Part model, mm, in its own coordinate system. Face numbers are marked on the shaded views. A direction names the side the tool comes from. Round coordinates to 2 decimals unless told otherwise and drop trailing zeros. Loops run counter-clockwise (first coordinate to the right, second up) from the corner with the lowest first, then second, coordinate; pieces in that order, holes last. Notation, with made-up numbers: M 61,37.25 L 75,37.25 A14 ccw 75,59.25 Z; hole C 22,-33 d10. An arc over 180 degrees is marked long. Answer as CSV lines item,"result". Start each with the question number.
Item 1: Mould opens along X. For the marked faces 1, 2, 3 and 4 say: pulls with the +X half, pulls with the -X half, needs draft (parallel to the pull), parting line crosses it, or undercut.
Item 2: Drop flat-ended pins along their axis: pin 1 Ø7.5 at (x, y) = (16, 4) entering from -Z; pin 2 Ø5.5 at (y, z) = (7.5, 9) entering from +X; pin 3 Ø5 at (x, y) = (23, 2.5) entering from +Z; pin 4 Ø2 at (x, z) = (24, 12) entering from -Y. Give the stop position or say it passes through.
Item 3: Band-saw the part on C-C (x = 25.25). Give the cut face in (y, z), and give its area (3 significant figures).
Item 4: Band-saw the part on B-B (y = 11.5). Give the cut face in (x, z).
Item 5: Band-saw the part on A-A (z = 3). Give the cut face in (x, y), and give its area (3 significant figures).
Item 6: Which spindle directions (+Z, -Z, +X, -X, +Y, -Y) get a long thin tool onto all of the face, cutting with end or side? Do the marked faces 5 and 6. Say none if no direction does.
Item 7: Band-saw the part on D-D (z = 9.75). Give the cut face in (x, y).
Item 8: Wall check: line 1 (X direction, y = 0.5, z = 2.5); line 2 (X direction, y = 11, z = 9); line 3 (Z direction, x = 11, y = 1.75). Give the ranges that are in metal, low to high.
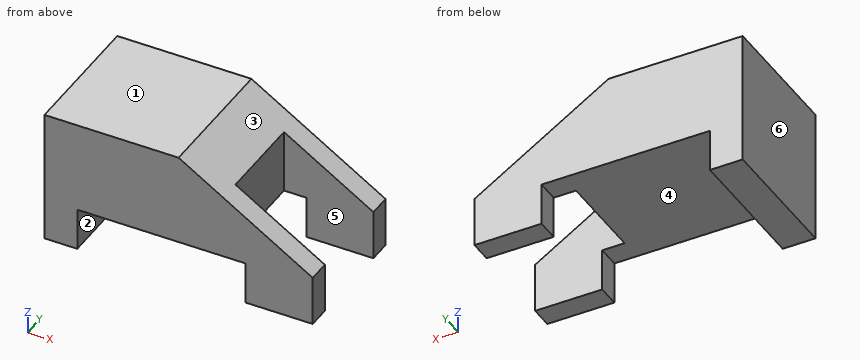
```python
from build123d import *

# Parameters (mm, degrees)
F1_DEPTH = 15
F3_DEPTH = 15.001
F2_W     = 18.829098
F2_H     = 4.753366
F4_DEPTH = 15.001


with BuildPart() as f1:
    # F0 (on Top) → F1 (new body)
    with BuildSketch(Plane.XY):
        Polygon((0, 15), (0, 0), (30, 0), (30, 2.5), (20, 2.5), (20, 12.5), (30, 12.5), (30, 15), align=None)
    extrude(amount=F1_DEPTH)

    # F2 (on face) → F3 (cut, through all)
    with BuildSketch(Plane.XZ):
        Polygon((30, 15), (15, 15), (30, 5.606282), align=None)
    extrude(amount=-F3_DEPTH, mode=Mode.SUBTRACT)

    # F2 (on face) → F4 (cut, through all)
    with BuildSketch(Plane.XZ):
        with Locations((13.085451, 2.376683)):
            Rectangle(F2_W, F2_H)
    extrude(amount=-F4_DEPTH, mode=Mode.SUBTRACT)


solid = f1.part
```
Answer block:
1,face 1,"needs draft"
1,face 2,"undercut"
1,face 3,"pulls with the +X half"
1,face 4,"undercut"
2,pin 1,"stops at z = 4.75"
2,pin 2,"stops at x = 20"
2,pin 3,"stops at z = 11.56"
2,pin 4,"passes through"
3,outline,"M 0,0 L 2.5,0 L 2.5,8.58 L 0,8.58 Z; M 12.5,0 L 15,0 L 15,8.58 L 12.5,8.58 Z"
3,area,"42.9 mm^2"
4,outline,"M 0,0 L 3.67,0 L 3.67,4.75 L 20,4.75 L 20,11.87 L 15,15 L 0,15 Z"
5,outline,"M 0,0 L 3.67,0 L 3.67,15 L 0,15 Z; M 22.5,0 L 30,0 L 30,2.5 L 22.5,2.5 Z; M 22.5,12.5 L 30,12.5 L 30,15 L 22.5,15 Z"
5,area,"92.6 mm^2"
6,face 5,"+Z, -Z, +X"
6,face 6,"+Z, -Z, -X, +Y, -Y"
7,outline,"M 0,0 L 23.38,0 L 23.38,2.5 L 20,2.5 L 20,12.5 L 23.38,12.5 L 23.38,15 L 0,15 Z"
8,line 1,"x = 0 to 3.67, 22.5 to 30"
8,line 2,"x = 0 to 20"
8,line 3,"z = 4.75 to 15"
